Could you check a few things on this model? Use its own coordinates, in mm. A direction names the side the tool comes from. Round coordinates to 2 decimals unless told otherwise and drop trailing zeros. Loops run counter-clockwise (first coordinate to the right, second up) from the corner with the lowest first, then second, coordinate; pieces in that order, holes last. Notation, with made-up numbers: (-9, -28.5) -> (32, -28.5) arc R16 ccw to (32, -20.5) -> close; hole circle Ø10 at (-38.75, 47). An arc over 180 degrees is marked (long way). One line per item, written item: value.
```python
from build123d import *

# Parameters (mm, degrees)
F1_ANGLE = 90
F2_DEPTH = 60
F4_DEPTH = 150


with BuildPart() as f1:
    # F0 (on Front) → F1 (revolve)
    with BuildSketch(Plane.XZ):
        Polygon((-0.0259582262, -11.9999719237), (10.3793014176, -6.0224664452), (10.4052596438, 5.9775054785), (0.0259582262, 11.9999719237), (-10.3793014176, 6.0224664452), (-10.4052596438, -5.9775054785), align=None)
    revolve(axis=Axis((-10.4052596438, 0, 8.529782465), (0, 0, -1)), revolution_arc=F1_ANGLE)

    # F0 (on Front) → F2 (join)
    with BuildSketch(Plane.XZ):
        Polygon((-0.0259582262, -11.9999719237), (10.3793014176, -6.0224664452), (10.4052596438, 5.9775054785), (0.0259582262, 11.9999719237), (-10.3793014176, 6.0224664452), (-10.4052596438, -5.9775054785), align=None)
    extrude(amount=-F2_DEPTH)

    # F3 (on face) → F4 (join)
    with BuildSketch(Plane(origin=(-10.4052596438, 0, 0), x_dir=(0, -1, 0), z_dir=(-1, 0, 0))):
        Polygon((0, -5.9775054785), (10.3793014176, -11.9999719237), (20.7845610613, -6.0224664452), (20.8105192875, 5.9775054785), (10.43121787, 11.9999719237), (0.0259582262, 6.0224664452), align=None)
    extrude(amount=F4_DEPTH)


solid = f1.part
```
(1) For pin 1 Ø1 at (x, y) = (-31, -5.5) entering from +Z; pin 2 Ø5 at (x, z) = (-43, -6.5) entering from -Y; pin 3 Ø2 at (y, z) = (14, -8) entering from +X, each with a flat end and sliding along its axis, tell me the tip position at first contact or that it passes through.
Results below:
pin 1: stops at z = 9.45
pin 2: stops at y = -20.79
pin 3: stops at x = 8.68
(2) On a 3-axis mill with a long thin cutter (end or side, diameter ignored), from which of +Z, -Z, +X, -X, +Y, -Y can I reach the whole of each face in a straight line? I mean faces 1 (the face through (-5.288, 29.58, -8.947)), 2 (the face through (-5.104, 29.58, 9.053)), 3 (the face through (-84.355, -15.509, -9.053)). Say none if no direction works.
Results below:
face 1: -Z, -X, +Y
face 2: +Z, -X, +Y
face 3: -Z, +X, -X, -Y
(3) Imagine slicing it at C-C on x = -52.5. Write out the boundary of the cut face in (y, z).
Results below:
outline: (-20.81, 5.98) -> (-20.78, -6.02) -> (-10.38, -12) -> (0, -5.98) -> (-0.03, 6.02) -> (-10.43, 12) -> close
(4) Imagine slicing it at A-A on y = 39.5. Write out the boundary of the cut face in (x, z).
Results below:
outline: (-10.41, -5.98) -> (-0.03, -12) -> (10.38, -6.02) -> (10.41, 5.98) -> (0.03, 12) -> (-10.38, 6.02) -> close
(5) Please list where these lines run through material, in increasing order: L1, parallel to Y at x = -81, z = -1.25; L2, parallel to X at y = 19.5, z = -4.75; L3, parallel to Z at x = -10, y = 17.
Results below:
L1: y = -20.79 to -0.01
L2: x = -10.4 to 10.38
L3: z = -6.21 to 6.24
